Autodesk Inventor part; units mm, degrees
ref_plane "YZ Plane" through (0, 0, 0) normal (1, 0, 0) x (0, 1, 0)
ref_plane "XZ Plane" through (0, 0, 0) normal (0, 1, 0) x (-1, 0, 0)
ref_plane "XY Plane" through (0, 0, 0) normal (0, 0, 1) x (1, 0, 0)
sketch "Sketch_base" plane through (0, 0, 0) normal (0, 0, 1) x (1, 0, 0)
  line L0 (0, 129.9853) -> (0, -82.9142) construction
  line L1 (-53.9995, 0) -> (53.9995, 0) construction
  line L2 (-36.5, 37.5) -> (36.5, 37.5)
  line L3 (36.5, 37.5) -> (36.5, -37.5)
  line L4 (36.5, -37.5) -> (-36.5, -37.5)
  line L5 (-36.5, -37.5) -> (-36.5, 37.5)
  line L6 (-36.5, 37.5) -> (36.5, -37.5) construction
  line L7 (36.5, 37.5) -> (-36.5, -37.5) construction
  line L8 (-35, -37.5) -> (35, -37.5)
  line L9 (35, -37.5) -> (35, -52.5)
  line L10 (35, -52.5) -> (-35, -52.5)
  line L11 (-35, -52.5) -> (-35, -37.5)
  line L12 (-35, -37.5) -> (35, -52.5) construction
  line L13 (35, -37.5) -> (-35, -52.5) construction
  line L14 (-26.5, 97.5) -> (26.5, 97.5)
  line L15 (36.5, 87.5) -> (36.5, 37.5)
  line L16 (36.5, 37.5) -> (-36.5, 37.5)
  line L17 (-36.5, 37.5) -> (-36.5, 87.5)
  line L18 (-36.5, 97.5) -> (36.5, 37.5) construction
  line L19 (36.5, 97.5) -> (-36.5, 37.5) construction
  arc A0 (-26.5, 97.5) -> (-36.5, 87.5) centre (-26.5, 87.5) ccw
  arc A1 (36.5, 87.5) -> (26.5, 97.5) centre (26.5, 87.5) ccw
  circle A2 centre (-30.5, 12.2) radius 1.6
  circle A3 centre (30.5, 12.2) radius 1.6
  circle A4 centre (16.2, -9.6) radius 2.5
  circle A5 centre (22.3, -9.6) radius 2.5
  circle A6 centre (28.6, -9.6) radius 2.5
  circle A7 centre (-31.5, -32) radius 1.6
  circle A8 centre (31.5, -32) radius 1.6
  circle A9 centre (-28, -12.5) radius 2.5
  point P0 (0, 0)
  point P1 (-20, -45.5)
  point P2 (20, -45.5)
  point P3 (0, -45)
  point P4 (0, 67.5)
  point P5 (-18, 87.5)
  point P6 (18, 87.5)
  point P7 (31.5, -32)
  dimension "d0" = 73
  dimension "d1" = 75
  dimension "d3" = 40
  dimension "d4" = 20
  dimension "d38" = 15
  dimension "d39" = 0
  dimension "d40" = 70
  dimension "d46" = 7
  dimension "d47" = 7
  dimension "d55" = 60
  dimension "d56" = 10
  dimension "d57" = 10
  dimension "d58" = 36
  dimension "d59" = 18
  dimension "d102" = 5.5
  dimension "d103" = 5.5
  dimension "d104" = 63
  dimension "d105" = 31.5
  dimension "d113" = 10
  dimension "d114" = 10
extrude "Plate1" add sketch "Sketch_base" along normal blind 1.5 contours L2 L3 L4 L5 | A2 | A3 | A4 | A5 | A6 | A7 | A8 | A9
sheet face with bend "Face2" sketch "Sketch_base" thickness 1.5 toward (0, 0, 1) bend radius 1.5 contours L4 L9 L10 L11
bend "Bend3"
hole "Hole2" at (-20, -45.5, 0) at (20, -45.5, 0) direction (0, 0, 1) diameter 6 end through all
sheet face with bend "Face3" sketch "Sketch_base" thickness 1.5 toward (0, 0, 1) bend radius 1.5 contours L17 A0 L14 A1 L15 L2
bend "Bend4"
hole "Hole3" at (18, 87.5, 0) at (-18, 87.5, 0) direction (0, 0, 1) diameter 10 end through all
sketch "Sketch4" plane through (-36.5, -37.5, 1.5) normal (-1, 0, 0) x (0, -1, 0)
  line L0 (-115, 0) -> (0, 0)
  line L1 (0, 0) -> (0, 18.5)
  line L2 (0, 18.5) -> (-115, 18.5)
  line L3 (-115, 18.5) -> (-115, 0)
edge flange "Flange3" height 20 angle 90 thickness 1.5 bend radius 1.5 thickness toward (-1, 0, 0) relief round relief width 1.5 relief depth 0.75 edges at (-36.5, 25, 1.5) wall of the first edge with corners at (-36.5, 77.5, 1.5) (-36.5, -37.5, 1.5) (-36.5, -37.5, 20) (-36.5, 77.5, 20)
bend "Bend5"
corner "Corner3"
sketch "Sketch5" plane through (36.5, 87.5, 1.5) normal (1, 0, 0) x (0, 1, 0)
  line L0 (-125, 0) -> (-10, 0)
  line L1 (-10, 0) -> (-10, 18.5)
  line L2 (-10, 18.5) -> (-125, 18.5)
  line L3 (-125, 18.5) -> (-125, 0)
edge flange "Flange4" height 20 angle 90 thickness 1.5 bend radius 1.5 thickness toward (1, 0, 0) relief round relief width 1.5 relief depth 0.75 edges at (36.5, 25, 1.5) wall of the first edge with corners at (36.5, -37.5, 1.5) (36.5, 77.5, 1.5) (36.5, 77.5, 20) (36.5, -37.5, 20)
bend "Bend6"
corner "Corner4"
sketch "Sketch6" plane through (-38, -37.5, 20) normal (-1, 0, 0) x (0, 0, 1)
  line L0 (0, 0) -> (0, 115)
  line L1 (0, 115) -> (-15, 115)
  line L2 (-15, 115) -> (-15, 65)
  line L3 (-15, 65) -> (0, 65)
  line L4 (0, 65) -> (0, 115)
  point P0 (-20, 37.5)
  point P1 (0, 65)
  dimension "d96" = 15
  dimension "d97" = 50
extrude "Extrusion1" cut sketch "Sketch6" against normal through all
fillet "Fillet1" radius 2 6 edges at (-37.25, 77.5, 5) (37.25, 77.5, 5) (37.25, 27.5, 20) (37.25, 27.5, 5) (-37.25, 27.5, 5) (-37.25, 27.5, 20)
fillet "Fillet2" radius 2 2 edges at (37.25, -37.5, 20) (-37.25, -37.5, 20)
hole "Hole4" at (-31.5, -32, 0) at (31.5, -32, 0) direction (0, 0, 1) diameter 3.2 end through all
fillet "Corner Round1" radius 2 2 edges at (-35, -52.5, 0.75) (35, -52.5, 0.75)
hole "Hole5" at (-30.5, 12.2, 0) at (30.5, 12.2, 0) direction (0, 0, 1) diameter 3.2 end through all
hole "Hole6" at (16.2, -9.6, 0) at (22.3, -9.6, 0) at (28.6, -9.6, 0) at (-28, -12.5, 0) direction (0, 0, 1) diameter 5 end through all
equation "\"d111\" = Thickness"
equation "\"d121\" = Thickness"
equation "\"d2\" = Thickness"
equation "\"d41\" = BendRadius"
equation "\"d42\" = BendReliefWidth"
equation "\"d44\" = MinimumRemnant"
equation "\"d43\" = BendReliefDepth"
equation "\"d45\" = TransitionRadius"
equation "\"d60\" = BendRadius"
equation "\"d61\" = BendReliefWidth"
equation "\"d63\" = MinimumRemnant"
equation "\"d62\" = BendReliefDepth"
equation "\"d64\" = TransitionRadius"
equation "\"d72\" = BendReliefWidth"
equation "\"d73\" = BendReliefDepth"
equation "\"d74\" = MinimumRemnant"
equation "\"d75\" = TransitionRadius"
equation "\"d78\" = BendRadius"
equation "\"d79\" = CornerReliefSize"
equation "\"d80\" = GapSize"
equation "\"d81\" = JacobiRadiusSize"
equation "\"d84\" = BendReliefWidth"
equation "\"d85\" = BendReliefDepth"
equation "\"d86\" = MinimumRemnant"
equation "\"d87\" = TransitionRadius"
equation "\"d92\" = BendRadius"
equation "\"d93\" = CornerReliefSize"
equation "\"d94\" = GapSize"
equation "\"d95\" = JacobiRadiusSize"
equation "\"BendRadius\" = Thickness"
equation "\"BendReliefWidth\" = Thickness"
equation "\"BendReliefDepth\" = 0.5 * Thickness"
equation "\"CornerReliefSize\" = 4 * Thickness"
equation "\"MinimumRemnant\" = 2 * Thickness"
equation "\"TransitionRadius\" = BendRadius"
equation "\"JacobiRadiusSize\" = BendRadius"
equation "\"GapSize\" = Thickness"
properties part number "Enclosure_Base"
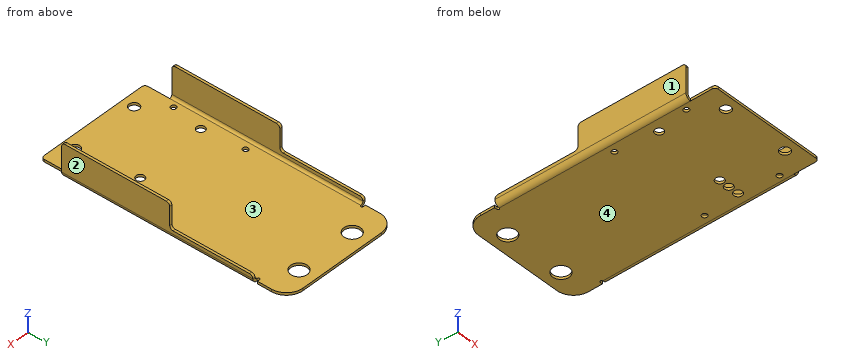
Read the model definition and answer for the solid it produces. Units are mm, in the model's axes. Face numbers are marked on the shaded views. Give positions to 0.01 mm unless a question says otherwise; leave off trailing zeros. Write each loop counter-clockwise with the first axis right and the second up, starting at its lowest first coordinate (ties: lowest second). Pieces come first, ordered by that corner, then holes. Notation, with made-up numbers: (14, -3.5) - (62, -3.5) arc R25 ccw to (62, 26.5) - close; hole circle Ø5 at (79, 29.5). An arc over 180 degrees is marked (long way). Answer in a Markdown table with one row per item. Add a question column.
Item 1: Determine the mould class of the marked faces 1, 2, 3 and 4 for opening direction X: pulls with the +X half, pulls with the -X half, needs draft (parallel to the pull), parting line crosses it, or undercut.
Item 2: Find the intervals of material crossed by L1, parallel to X at y = -32, z = 0.4; L2, parallel to X at y = -45.5, z = 0.9; L3, parallel to X at y = -30, z = 19.25, in increasing order.
Item 3: Section D-D, the plane x = 3.5 is taken. Write down the section's boundary in (y, z), and give its area (3 significant figures).
Item 4: Section A-A, the plane z = 10.75 is taken. Write down the section's boundary in (x, y), and give its area (3 significant figures).
Item 5: Flat-ended cylindrical pins translate along their axes: P1, Ø6, axis at y = 44, z = 7, coming from the -X side; P2, Ø1.5, axis at x = 29, y = 8, coming from the +Z side; P3, Ø3.5, axis at x = 36, z = 2, coming from the +Y side; P4, Ø0.8, axis at x = -37, z = 12.5, coming from the +Y side. Find the tip coordinate at first contact, or state that the pin passes through.
Item 6: Section C-C, the plane y = 9 is taken. Write down the section's boundary in (x, z).
Item 7: Section B-B, the plane y = 86 is taken. Write down the section's boundary in (x, z), and give its area (3 significant figures).
Recorded:
| question | item | result |
|---|---|---|
| 1 | face 1 | pulls with the -X half |
| 1 | face 2 | pulls with the +X half |
| 1 | face 3 | undercut |
| 1 | face 4 | needs draft |
| 2 | L1 | x = -36.5 to -33.1, -29.9 to 29.9, 33.1 to 36.5 |
| 2 | L2 | x = -35 to -23, -17 to 17, 23 to 35 |
| 2 | L3 | x = -38 to -36.5, 36.5 to 38 |
| 3 | outline | (-52.5, 0) - (97.5, 0) - (97.5, 1.5) - (-52.5, 1.5) - close |
| 3 | area | 225 mm2 |
| 4 | outline | (-38, -37.5) - (-36.5, -37.5) - (-36.5, 27.5) - (-38, 27.5) - close; (36.5, -37.5) - (38, -37.5) - (38, 27.5) - (36.5, 27.5) - close |
| 4 | area | 195 mm2 |
| 5 | P1 | stops at x = -38 |
| 5 | P2 | stops at z = 1.5 |
| 5 | P3 | stops at y = 93.73 |
| 5 | P4 | stops at y = 27.5 |
| 6 | outline | (-38, 3) arc R3 ccw to (-35, 0) - (35, 0) arc R3 ccw to (38, 3) - (38, 20) - (36.5, 20) - (36.5, 3) arc R1.5 cw to (35, 1.5) - (-35, 1.5) arc R1.5 cw to (-36.5, 3) - (-36.5, 20) - (-38, 20) - close |
| 7 | outline | (-36.5, 0) - (-22.77, 0) - (-22.77, 1.5) - (-36.5, 1.5) - close; (-13.23, 0) - (13.23, 0) - (13.23, 1.5) - (-13.23, 1.5) - close; (22.77, 0) - (36.5, 0) - (36.5, 1.5) - (22.77, 1.5) - close |
| 7 | area | 80.9 mm2 |
